Input: part model. Units: mm. Frame: model coordinates. A direction names the side the tool comes from. Round coordinates to 2 decimals unless told otherwise and drop trailing zeros. Loops run counter-clockwise (first coordinate to the right, second up) from the corner with the lowest first, then second, coordinate; pieces in that order, holes last. Notation, with made-up numbers: (58.5, -17.5) -> (115.5, -17.5) arc R22 cw to (115.5, -9.5) -> close; hole circle Ø3 at (14, 88.25). An arc over 180 degrees is marked (long way). Answer in a Markdown table with one row per item. Add a question column.
Q1. Ray query, L1, parallel to X at y = 0.5, z = -88.5; L2, parallel to Y at x = 0, z = -118; L3, parallel to Z at x = 15, y = -9. Return the intervals inside material, ascending. Write a range as from..to.
Q2. Pin query (flat end, axial travel): pin 1 (12 mm diameter, centred on y = -7.5, z = -106, fed in from -X); pin 2 (18 mm diameter, centred on x = 0, y = 0, fed in from -Z); pin 3 (8 mm diameter, centred on y = -13.5, z = -41.5, fed in from +X); pin 4 (5 mm diameter, centred on x = 6.5, z = -68, fed in from -Y). Return the tip coordinate at first contact, or that it passes through.
Q3. Reachability of faces 4 (the face through (-2.94, 9.32, -11.99)), 5 (the face through (18.59, -2.44, -112.72)), 6 (the face through (-6, 4, -11)) from +Z, -Z, +X, -X, +Y, -Y: full face, straight path, thin tool, end or side. Return the list, or none.
Q4. Section A-A, the plane z = -61. Output: boundary loops of the cut face in (x, y), and give its area (3 significant figures).
Q5. Section B-B, the plane z = -33. Output: boundary loops of the cut face in (x, y), and give its area (3 significant figures).
Q6. Mould query, pull axis X, two halves, no side actions, for faces 1 (the face through (0, -12, 0)), 2 (the face through (18.59, -2.44, -36.47)), 3 (the face through (3, 5.5, -116)). Classes: pulls with the +X half, pulls with the -X half, needs draft (parallel to the pull), parting line crosses it, or undercut.
Autodesk Inventor part; units mm, degrees
ref_plane "YZ Plane" through (0, 0, 0) normal (1, 0, 0) x (0, 1, 0)
ref_plane "XZ Plane" through (0, 0, 0) normal (0, 1, 0) x (-1, 0, 0)
ref_plane "XY Plane" through (0, 0, 0) normal (0, 0, 1) x (1, 0, 0)
sketch "Esquisse1" plane through (0, 0, 0) normal (1, 0, 0) x (0, 1, 0)
  line L0 (0, 0) -> (0, -31.2712)
  line L1 (18.75, -30) -> (18.75, -120)
  line L2 (18.75, -120) -> (0, -120)
  line L3 (14.75, -116) -> (14.75, -55.9524)
  line L4 (14.75, -55.9524) -> (7, -12)
  line L5 (7, -12) -> (7, -11)
  line L6 (7, -11) -> (8, -11)
  line L7 (8, -11) -> (9.7, -12.2)
  line L8 (9.7, -12.2) -> (10.85, -8.8246)
  line L9 (10.85, -8.8246) -> (8.25, -8)
  circle A0 centre (8.85, -9.7639) radius 1.5 construction
  line L10 (8.25, -8) -> (8.25, -7)
  line L11 (8.25, -7) -> (11.75, 0)
  line L12 (18.75, -30) -> (12.25, -30)
  line L13 (12.25, -30) -> (12.25, 0)
  line L14 (12.25, 0) -> (11.75, 0)
  line L15 (0, -120) -> (0, -116)
  line L16 (14.75, -116) -> (0, -116)
  point P0 (9.7477, -27.583)
  dimension "d1" = 37.5
  dimension "d3" = 14
  dimension "d6" = 3
  dimension "d7" = 1
  dimension "d8" = 1
  dimension "d11" = 3
  dimension "d12" = 0.6
  dimension "d13" = 1.2
  dimension "d14" = 1.7
  dimension "d15" = 2.6
  dimension "d29" = 24.5
  dimension "d30" = 0.5
  dimension "d31" = 30
  dimension "d34" = 1
  dimension "d36" = 16.5
  dimension "d37" = 11
  dimension "d38" = 90
  dimension "d58" = 7.75
  dimension "d59" = 170
  dimension "d60" = 19.4954
  dimension "d61" = 4
  dimension "d62" = 4
revolve "Révolution2" add sketch "Esquisse1" angle 360 about axis through (0, 0, 0) along (0, 0, -1)
sketch "Esquisse2" plane through (0, 0, 0) normal (0, 1, 0) x (-1, 0, 0)
  line L0 (-18.75, -30) -> (18.75, -30)
  line L1 (-18.75, -120) -> (18.75, -120)
  line L2 (-14.75, -55.9524) -> (14.75, -55.9524)
  line L3 (-7, -12) -> (7, -12)
  line L4 (-18.75, -30) -> (-18.75, -120)
  line L5 (-18.75, -42.7677) -> (-16.25, -41.8578)
  line L6 (-16.25, -41.8578) -> (-16.25, -46.1422)
  line L7 (-16.25, -46.1422) -> (-18.75, -45.2323)
  circle A0 centre (-17.75, -44) radius 1.5 construction
  line L8 (0, -144) -> (0, 24)
  point P0 (0, 0)
  dimension "d42" = 3
  dimension "d45" = 1
  dimension "d46" = 70
  dimension "d47" = 70
  dimension "d48" = 14
revolve "Révolution3" cut sketch "Esquisse2" angle 360 about axis through (0, 0, -10) along (0, 0, 1) contours L5 L6 L7 L4
chamfer "Chanfrein4" distance 1.5 angle 45 1 edges at (0, -12.25, -30)
pattern_linear "Réseau rectangulaire1" count 2 spacing 60 along (0, 0, -1) of "Révolution3"
chamfer "Chanfrein5" distance 2 angle 45 1 edges at (0, -14.75, -116)
sketch "Esquisse3" plane through (0, 0, 0) normal (0, 0, 1) x (1, 0, 0)
  circle A0 centre (0, 0) radius 11.75
  circle A1 centre (0, 0) radius 12.25
  line L0 (-1, 14.2091) -> (1, 14.2091)
  line L1 (1, 14.2091) -> (1, 12.2091)
  line L2 (1, 12.2091) -> (-1, 12.2091)
  line L3 (-1, 12.2091) -> (-1, 14.2091)
  circle A2 centre (0, 0) radius 12.25
  point P0 (0, 12.2091)
  dimension "d66" = 2
  dimension "d67" = 2
extrude "Extrusion1" add sketch "Esquisse3" against normal up to surface (30 mm away) contours L2 A1 | A1 L3 L0 L1 picked at (-0.1112, 12.2212)
chamfer "Chanfrein6" distance 0.5 angle 45 2 edges at (1, 14.2091, -15) (-1, 14.2091, -15)
sketch "Esquisse8" plane through (0, 0, -120) normal (0, 0, -1) x (-1, 0, 0)
  circle A0 centre (0, 0) radius 5
  dimension "d100" = 10
extrude "Extrusion5" cut sketch "Esquisse8" against normal up to surface (4 mm away)
chamfer "Chanfrein8" distance 1 angle 45 2 edges at (5, 0, -120) (5, 0, -116)
sketch "Esquisse9" plane through (0, 0, 0) normal (0, 1, 0) x (-1, 0, 0)
  line L0 (1, 0) -> (1, -28.5)
  line L1 (-1, -28.5) -> (1, -28.5)
  line L2 (-1, -28.5) -> (-1, 0)
  line L3 (-1, 0) -> (1, 0)
  line L4 (8.25, -7) -> (11.75, 0)
  line L5 (-8.25, -7) -> (-11.75, 0)
  line L6 (12.25, 0) -> (-12.25, 0)
  line L7 (-12.25, 0) -> (-12.25, -5)
  line L8 (-12.25, -5) -> (12.25, -5)
  line L9 (12.25, -5) -> (12.25, 0)
  line L10 (-12.25, 0) -> (12.25, 0)
  line L11 (-8.25, -7) -> (8.25, -7)
  line L12 (-12.25, 0) -> (-12.25, -28.5)
  point P0 (0, 0)
  dimension "d108" = 2
  dimension "d112" = 5
extrude "Extrusion6" cut sketch "Esquisse9" along normal blind 15 contours L6 L4 L8 L0 | L0 L8 L2 L3 | L2 L8 L5 L6 | L6 L9 L8 L4 | L5 L8 L7 L6
chamfer "Chanfrein9" distance 2 angle 45 2 edges at (10.5, 0, -2.5) (-10.5, 0, -2.5)
equation "\"d47\" = d46"
properties part number "douille_bloqueur"
Answer block:
| question | item | result |
|---|---|---|
| 1 | L1 | -18.74..-14.74, 14.74..18.74 |
| 1 | L2 | -18.75..-5, 5..18.75 |
| 1 | L3 | -120..-105.69, -102.31..-45.69, -42.31..-30 |
| 2 | pin 1 | x = -18.69 |
| 2 | pin 2 | z = -120 |
| 2 | pin 3 | x = 16.17 |
| 2 | pin 4 | y = -18.32 |
| 3 | face 4 | none |
| 3 | face 5 | +Z, -Z |
| 3 | face 6 | +Z |
| 4 | outline | circle Ø37.5 at (0, 0); hole circle Ø29.5 at (0, 0) |
| 4 | area | 421 mm^2 |
| 5 | outline | circle Ø37.5 at (0, 0); hole circle Ø21.41 at (0, 0) |
| 5 | area | 745 mm^2 |
| 6 | face 1 | needs draft |
| 6 | face 2 | parting line crosses it |
| 6 | face 3 | undercut |
